Verification items for the finished model (mm, model axes). A direction names the side the tool comes from. Coordinates: 2 decimals unless noted, no trailing zeros. Order: outer loops, then holes, each group sorted by start corner. A loop starts at its lowest first (then second) coordinate and runs counter-clockwise, first axis right, second up. Notation, with made-up numbers: (8, 59) -> (63, 59) arc R26 cw to (63, 90) -> close; hole circle Ø3 at (13.25, 28). An arc over 180 degrees is marked (long way). Answer as CSV lines item,"result".
```python
from build123d import *

# Parameters (mm, degrees)
SKETCH1_R           = 23.5
BOSS_EXTRUDE1_DEPTH = 4
SKETCH2_R           = 23.5
BOSS_EXTRUDE2_DEPTH = 6


with BuildPart() as part:
    # Sketch1 → Boss-Extrude1 (new body)
    with BuildSketch(Plane.XY):
        Polygon((34.641016151, 20), (0, 40), (-34.641016151, 20), (-34.641016151, -20), (0, -40), (34.641016151, -20), align=None)
        Circle(SKETCH1_R, mode=Mode.SUBTRACT)
    extrude(amount=BOSS_EXTRUDE1_DEPTH)

    # Sketch2 → Boss-Extrude2 (add)
    with BuildSketch(Plane.XY):
        Circle(SKETCH2_R)
    extrude(amount=BOSS_EXTRUDE2_DEPTH)


solid = part.part
```
Item 1: Depth check by flat-ended pin: pin 1 Ø2 at (y, z) = (-25.5, 1) entering from +X; pin 2 Ø3 at (x, y) = (-24, -9) entering from +Z; pin 3 Ø1.5 at (x, z) = (10.5, 2.5) entering from +Y. Enter the tip coordinate at first touch or a pass-through.
Answer list:
pin 1,"x = 26.85"
pin 2,"z = 4"
pin 3,"y = 34.37"
Item 2: Section check A-A, the plane y = 0. Record the boundary of the cut face in (x, z).
Answer list:
outline,"(-34.64, 0) -> (34.64, 0) -> (34.64, 4) -> (23.5, 4) -> (23.5, 6) -> (-23.5, 6) -> (-23.5, 4) -> (-34.64, 4) -> close"
Item 3: Section check C-C, the plane x = -3.5. Record the boundary of the cut face in (y, z).
Answer list:
outline,"(-37.98, 0) -> (37.98, 0) -> (37.98, 4) -> (23.24, 4) -> (23.24, 6) -> (-23.24, 6) -> (-23.24, 4) -> (-37.98, 4) -> close"
Item 4: Section check B-B, the plane z = 2.55. Record the boundary of the cut face in (x, y).
Answer list:
outline,"(-34.64, -20) -> (0, -40) -> (34.64, -20) -> (34.64, 20) -> (0, 40) -> (-34.64, 20) -> close"
Item 5: Thickness scan on line 1 (Z direction, x = 21, y = 11.5); line 2 (Y direction, x = -13.5, z = 1.5); line 3 (Y direction, x = 1, z = 2.45). Record the ranges inside material, lowest first.
Answer list:
line 1,"0 to 4"
line 2,"-32.21 to 32.21"
line 3,"-39.42 to 39.42"
Item 6: Section check D-D, the plane y = -32.5. Record the boundary of the cut face in (x, z), plus the area to 3 significant figures.
Answer list:
outline,"(-12.99, 0) -> (12.99, 0) -> (12.99, 4) -> (-12.99, 4) -> close"
area,"104 mm2"
Item 7: Tool access check on faces 1 (the flat face through (34.641, 0, 2)), 2 (the cylindrical face through (22.4, 7.1, 5)). Record the directions out of +Z, -Z, +X, -X, +Y, -Y that give a thin tool (end or side, any length) a straight path to the whole face; none if there is none.
Answer list:
face 1,"+Z, -Z, +X, +Y, -Y"
face 2,"+Z"
